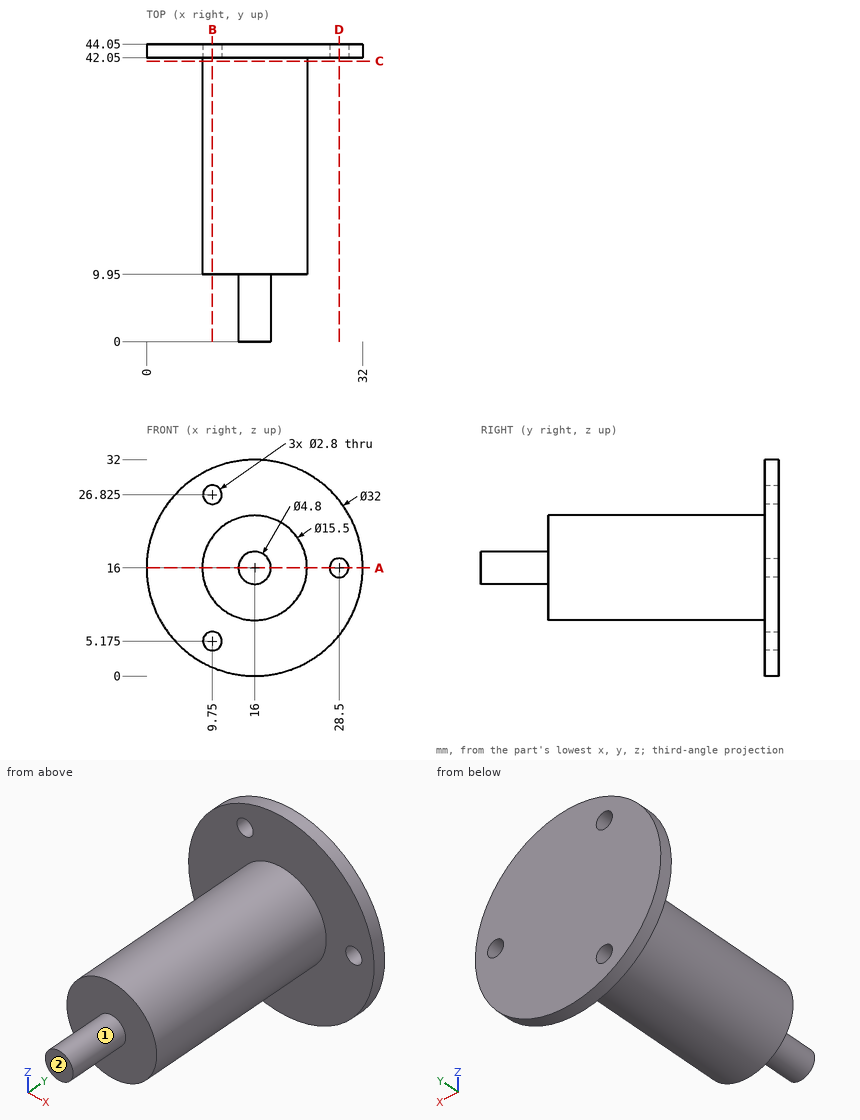
Geometry: see drawing. Coordinates: mm, zero at the bounding-box minimum. A direction names the side the tool comes from. Give positions to 0.01 mm unless a question says otherwise; leave off trailing zeros. Loops run counter-clockwise (first coordinate to the right, second up) from the corner with the lowest first, then second, coordinate; pieces in that order, holes last. Notation, with made-up numbers: (-15.5, 37) -> (32.5, 37) arc R12 cw to (32.5, 49) -> close; hole circle Ø8 at (49.5, 17.5). An arc over 180 degrees is marked (long way). Put each result on its own line as item: value.
1. Cut plane C-C (y = 41.5). Return the cut outline in (x, z), plus the area to 3 significant figures.
Taken from the geometry:
outline: circle Ø15.5 at (16, 16)
area: 189 mm2
2. Cut plane D-D (x = 28.5). Return the cut outline in (y, z).
Taken from the geometry:
outline: (42.05, 6.01) -> (44.05, 6.01) -> (44.05, 14.6) -> (42.05, 14.6) -> close; (42.05, 17.4) -> (44.05, 17.4) -> (44.05, 25.99) -> (42.05, 25.99) -> close
3. Cut plane B-B (x = 9.75). Count the separate pieces of the cut face and the enclosed holes in it, plus the area to 3 significant figures.
Taken from the geometry:
separate pieces: 3
enclosed holes: 0
area: 342 mm2
4. Ray query, line 1 along Z through (x, y) = (9.75, 42.9) (1 decimal); line 2 along Y through (x, z) = (26.5, 23); line 3 along Y through (x, z) = (18, 21). Return the intervals inside material, ascending. Write a range as [from, to].
Taken from the geometry:
line 1: z = [1.3, 3.8], [6.6, 25.4], [28.2, 30.7]
line 2: y = [42.05, 44.05]
line 3: y = [9.95, 44.05]
5. Cut plane A-A (z = 16). Return the cut outline in (x, y).
Taken from the geometry:
outline: (0, 42.05) -> (8.25, 42.05) -> (8.25, 9.95) -> (13.6, 9.95) -> (13.6, 0) -> (18.4, 0) -> (18.4, 9.95) -> (23.75, 9.95) -> (23.75, 42.05) -> (27.1, 42.05) -> (27.1, 44.05) -> (0, 44.05) -> close; (29.9, 42.05) -> (32, 42.05) -> (32, 44.05) -> (29.9, 44.05) -> close
6. Set-up query: the marked faces 1 and 2. Return all of +Z, -Z, +X, -X, +Y, -Y with unobstructed straight access to the full face (end or side cutting, diameter ignored); none if empty.
Taken from the geometry:
face 1: -Y
face 2: +Z, -Z, +X, -X, -Y
7. Pin query (flat end, axial travel): P1, Ø2.5, axis at x = 9.75, z = 5.17, coming from the -Y side; P2, Ø3, axis at y = 30, z = 8.5, coming from the -X side (1 decimal); P3, Ø1, axis at x = 11, y = 32, coming from the -Z side; P4, Ø5, axis at y = 11.5, z = 9, coming from the +X side. Return the tip coordinate at first contact, or that it passes through.
Taken from the geometry:
P1: passes through
P2: stops at x = 11.1
P3: stops at z = 9.69
P4: stops at x = 22.31
